```python
from build123d import *

# Parameters (mm, degrees)
F1_DEPTH = 3


with BuildPart() as f1:
    # F0 (on Front) → F1 (new body)
    with BuildSketch(Plane.XZ):
        with BuildLine():
            Line((0, -5.363059), (0, 29.916195))
            Line((0, 29.916195), (-14.000191, 29.916195))
            Line((-14.000191, 29.916195), (-26.837912, 11.658107))
            ThreePointArc((-26.837912, 11.658107), (-26.839461, 12.040159), (-26.849809, 12.422075))
            ThreePointArc((-26.849809, 12.422075), (-43.382305, 11.673262), (-30.923461, 22.566442))
            Line((-30.923461, 22.566442), (-30.782148, 22.815704))
            ThreePointArc((-30.782148, 22.815704), (-60.191077, 11.081451), (-29.905884, 1.841057))
            Line((-29.905884, 1.841057), (-13.883179, -5.363059))
            Line((-13.883179, -5.363059), (0, -5.363059))
        make_face()
    extrude(amount=F1_DEPTH)


solid = f1.part
```
Work out the finished part from the listing and answer in its coordinate system (mm). A direction names the side the tool comes from. Give positions to 0.01 mm unless a question says otherwise; leave off trailing zeros. Order: outer loops, then holes, each group sorted by start corner. A loop starts at its lowest first (then second) coordinate and runs counter-clockwise, first axis right, second up.
1. Section B-B, the plane z = 13 is taken. Determine the outline of the cut face in (x, y).
Result sheet:
outline: (-60.16, -3) - (-43.8, -3) - (-43.8, 0) - (-60.16, 0) - close; (-25.89, -3) - (0, -3) - (0, 0) - (-25.89, 0) - close
2. Section C-C, the plane x = -38 is taken. Determine the outline of the cut face in (y, z), and give its area (3 significant figures).
Result sheet:
outline: (-3, -4.1) - (0, -4.1) - (0, 6.62) - (-3, 6.62) - close; (-3, 23.26) - (0, 23.26) - (0, 27.66) - (-3, 27.66) - close
area: 45.3 mm2
3. Section D-D, the plane x = -53 is taken. Determine the outline of the cut face in (y, z).
Result sheet:
outline: (-3, -2) - (0, -2) - (0, 25.56) - (-3, 25.56) - close
4. Section A-A, the plane y = -2.35 is taken. Determine the outline of the cut face in (x, z).
Result sheet:
outline: (-30.92, 22.57) - (-30.78, 22.82) arc R16.78 ccw (long way) to (-29.91, 1.84) - (-13.88, -5.36) - (0, -5.36) - (0, 29.92) - (-14, 29.92) - (-26.84, 11.66) arc R16.59 ccw to (-26.85, 12.42) arc R8.77 cw (long way) to start
5. Straight lines are drawn through the part: L1, parallel to Z at x = -32, y = -2.35; L2, parallel to X at y = -2, z = -3; L3, parallel to Z at x = -21.5, y = -1.2. For each, find the intervals that lie inside material, in ascending order.
Result sheet:
L1: z = -0.51 to 6.8, 23.08 to 24.07
L2: x = -51.37 to -35.48, -19.14 to 0
L3: z = -1.94 to 19.25
6. The mould has two halves that part along X. Classify faces 1 (the flat face through (0, -1, 12)), 2 (the cylindrical face through (-60.205, -1.479, 11.661)), 3 (the flat face through (-22.01, -1.48, -1.71)), 4 (the flat face through (-7, -1, 29.916)): released by +X, released by -X, zero draft, split by the parting line, or undercut.
Result sheet:
face 1: released by +X
face 2: undercut
face 3: undercut
face 4: zero draft
7. For faces 5 (the flat face through (-7, -1, -5.363)), 6 (the flat face through (-20.329, -1.479, 20.915)), determine the directions among +Z, -Z, +X, -X, +Y, -Y from which every point of the face is accessible in a straight line to the end or side of a thin tool.
Result sheet:
face 5: -Z, +X, -X, +Y, -Y
face 6: +Z, +Y, -Y
